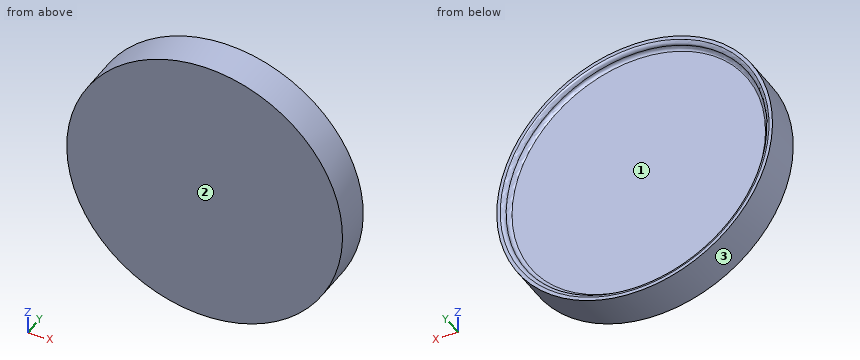
```python
from build123d import *

# Parameters (mm, degrees)
SKETCH1_R           = 457.2
BOSS_EXTRUDE1_DEPTH = 127
SKETCH2_R           = 433.036421312
CUT_EXTRUDE2_DEPTH  = 25.4
FILLET3_R           = 12.7
FILLET4_R           = 12.7


with BuildPart() as part:
    # Sketch1 → Boss-Extrude1 (new body)
    with BuildSketch(Plane(origin=(0, 0, 0), x_dir=(1, 0, 0), z_dir=(0, 1, 0))):
        with Locations(Location((0, 0, 0), (0, 0, 270))):
            Circle(SKETCH1_R)
    extrude(amount=BOSS_EXTRUDE1_DEPTH)

    # Sketch2 → Cut-Extrude2 (cut)
    with BuildSketch(Plane(origin=(0, 127, 0), x_dir=(1, 0, 0), z_dir=(0, 1, 0))):
        with Locations(Location((0, 0, 0), (0, 0, 270))):
            Circle(SKETCH2_R)
    extrude(amount=-CUT_EXTRUDE2_DEPTH, mode=Mode.SUBTRACT)

    # Fillet3
    fillet3_edges = [part.edges().sort_by_distance(p)[0] for p in [
        (0, 127, -433.036421312),
    ]]
    fillet(fillet3_edges, radius=FILLET3_R)

    # Fillet4
    fillet4_edges = [part.edges().sort_by_distance(p)[0] for p in [
        (0, 101.6, -433.036421312),
    ]]
    fillet(fillet4_edges, radius=FILLET4_R - 0.0001)  # a hair under: the kernel refuses the full size


solid = part.part
```
Read the model definition and answer for the solid it produces. Units are mm, in the model's axes. Face numbers are marked on the shaded views. Give positions to 0.01 mm unless a question says otherwise; leave off trailing zeros. Loops run counter-clockwise (first coordinate to the right, second up) from the corner with the lowest first, then second, coordinate; pieces in that order, holes last.
Item 1: The mould has two halves that part along Z. Classify the marked faces 1, 2 and 3: released by +Z, released by -Z, zero draft, split by the parting line, or undercut.
Item 2: Each of these flat-tipped pins is pushed along its axis until it touches: pin 1 Ø2 at (x, y) = (-171.5, 107.5) entering from +Z; pin 2 Ø12 at (x, y) = (194, 37.5) entering from +Z; pin 3 Ø5 at (y, z) = (98, 340) entering from +X. Where does it stop, or does it pass through?
Item 3: The part is cut by section C-C (y = 32.5). Write down the section's boundary in (x, z).
Item 4: Find the intervals of material crossed by line 1 along Y through (x, z) = (-222, -303.5); line 2 along X through (y, z) = (114.3, 0); line 3 along Y through (x, z) = (270, 336), in increasing order.
Taken from the geometry:
1. face 1: undercut
1. face 2: zero draft
1. face 3: split by the parting line
2. pin 1: stops at z = 424.22
2. pin 2: stops at z = 416.76
2. pin 3: stops at x = 308.42
3. outline: circle Ø914.4 at (0, 0)
4. line 1: y = 0 to 101.6
4. line 2: x = -457.2 to -433.04, 433.04 to 457.2
4. line 3: y = 0 to 107.47
